from build123d import *

# Parameters (mm, degrees)
SKETCH1_R               = 9
SKETCH1_R_2             = 5.9
BOSS_EXTRUDE1_DEPTH     = 23.8
CUT_EXTRUDE5_START      = 6.5
SKETCH3_R               = 7.65
CUT_EXTRUDE5_DEPTH      = 21.489627637
CUT_EXTRUDE6_DEPTH      = 30.7941271
CUT_EXTRUDE6_DEPTH_BACK = 7
SKETCH6_R               = 5.5
SKETCH7_R               = 13.484313598
CUT_EXTRUDE7_DEPTH      = 20.520246068


with BuildPart() as part:
    # Sketch1 → Boss-Extrude1 (new body)
    with BuildSketch(Plane(origin=(0, 0, 0), x_dir=(1, 0, 0), z_dir=(0, 1, 0))):
        with Locations(Location((0, 0, 0), (0, 0, 270))):
            Circle(SKETCH1_R)
        with Locations(Location((0, 0, 0), (0, 0, 270))):
            Circle(SKETCH1_R_2, mode=Mode.SUBTRACT)
    extrude(amount=-BOSS_EXTRUDE1_DEPTH)

    # Sketch3 → Cut-Extrude5 (cut, through all)
    with BuildSketch(Plane.XY.offset(CUT_EXTRUDE5_START)):
        with Locations((0, -8.4)):
            Circle(SKETCH3_R)
    extrude(amount=CUT_EXTRUDE5_DEPTH, mode=Mode.SUBTRACT)

    # Sketch6 → Cut-Extrude6 (cut, two sides: drawn at the far end of the back side and taken through both)
    with BuildSketch(Plane.XY.offset(6.5).offset(-CUT_EXTRUDE6_DEPTH_BACK)):
        with Locations(Location((0.145476138, -8.4, 0), (0, 0, 91.515662264))):
            Circle(SKETCH6_R)
    extrude(amount=CUT_EXTRUDE6_DEPTH + CUT_EXTRUDE6_DEPTH_BACK, mode=Mode.SUBTRACT)

    # Sketch7 → Cut-Extrude7 (cut, through all)
    with BuildSketch(Plane(origin=(0, -14.8, 0), x_dir=(-1, 0, 0), z_dir=(0, -1, 0))):
        Circle(SKETCH7_R)
    extrude(amount=-CUT_EXTRUDE7_DEPTH, mode=Mode.SUBTRACT)


solid = part.part
Here's how the part is built. I have some questions about the finished solid (model axes, mm). A direction names the side the tool comes from. Round coordinates to 2 decimals unless told otherwise and drop trailing zeros. Loops run counter-clockwise (first coordinate to the right, second up) from the corner with the lowest first, then second, coordinate; pieces in that order, holes last. Notation, with made-up numbers: M 58.25,-17 L 109.25,-17 A8 cw 109.25,-13 Z; hole C 71.5,54 d2. An arc over 180 degrees is marked long. Write each question's results on one line, items separated by ' | '. Start each with the question number.
(1) Thinking about a two-plate mould opening in X: for faces 1 (the cylindrical face through (0, -19, -9)), 2 (the flat face through (0, -15, 6.5)), 3 (the flat face through (0.1, -14.8, -6.3)), 4 (the cylindrical face through (-5.76, -19.24, -1.28)), which applies, pulls with the +X half, pulls with the -X half, needs draft (parallel to the pull), parting line crosses it, or undercut?
(2) I want a section at C-C (y = -18). Please give me the cut outline in (x, z), then the cut area to 3 significant figures.
(3) On a 3-axis mill with a long thin cutter (end or side, diameter ignored), from which of +Z, -Z, +X, -X, +Y, -Y can I reach the whole of each face in a straight line? I mean faces 5 (the cylindrical face through (-0.06, -16.05, 7.45)), 6 (the flat face through (-6, -23.8, 2)). Say none if no direction works.
(4) I want a section at A-A (z = 0). Please give me the cut outline in (x, y), then the cut area to 3 significant figures.
(5) If I drill on probe 1 along X at (y, z) = (-20, 0); probe 2 along X at (y, z) = (-22.75, 2.5); probe 3 along Z at (x, y) = (5, -23.25), over which ranges is the centre line in solid material (lowest first)? Write a range as from..to.
(6) Will these pins go through, and if not, where does the flat tip stop? P1, Ø1.5, axis at y = -20.5, z = 1.5, coming from the +X side; P2, Ø1.5, axis at y = -17.5, z = -7, coming from the -X side; P3, Ø5, axis at y = -16.5, z = 5, coming from the +X side.
(7) I want a section at D-D (x = 5). Please give me the cut outline in (y, z), then the cut area to 3 significant figures.
(8) I want a section at B-B (x = 0). Please give me the cut outline in (y, z), then the cut area to 3 significant figures.
Solved:
1) face 1: parting line crosses it | face 2: undercut | face 3: needs draft | face 4: undercut
2) outline: C 0,0 d18; hole C 0,0 d11.8 | area: 145 mm²
3) face 5: +Z, +Y | face 6: +Z, -Z, +X, -X, -Y
4) outline: M -9,-23.8 L -5.9,-23.8 L -5.9,-14.8 L -9,-14.8 Z; M 5.9,-23.8 L 9,-23.8 L 9,-14.8 L 5.9,-14.8 Z | area: 55.8 mm²
5) probe 1: x = -9..-5.9, 5.9..9 | probe 2: x = -8.65..-5.34, 5.34..8.65 | probe 3: z = -7.48..-3.13, 3.13..7.48
6) P1: stops at x = 8.97 | P2: stops at x = -6.48 | P3: stops at x = 8.65
7) outline: M -23.8,-7.48 L -14.8,-7.48 L -14.8,-3.13 L -23.8,-3.13 Z; M -23.8,3.13 L -14.8,3.13 L -14.8,7.48 L -23.8,7.48 Z | area: 78.3 mm²
8) outline: M -23.8,-9 L -14.8,-9 L -14.8,-5.9 L -23.8,-5.9 Z; M -23.8,5.9 L -14.8,5.9 L -14.8,6.5 L -16.05,6.5 L -16.05,9 L -23.8,9 Z | area: 52.7 mm²
